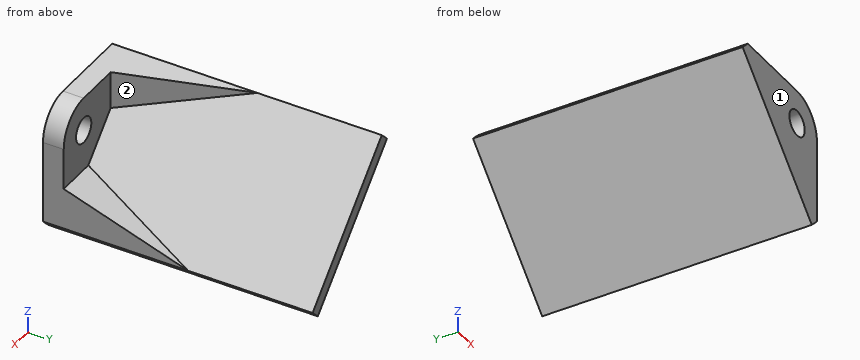
Autodesk Inventor part; units mm, degrees
ref_plane "YZ Plane" through (0, 0, 0) normal (1, 0, 0) x (0, 1, 0)
ref_plane "XZ Plane" through (0, 0, 0) normal (0, 1, 0) x (-1, 0, 0)
ref_plane "XY Plane" through (0, 0, 0) normal (0, 0, 1) x (1, 0, 0)
sketch "스케치1" plane through (0, 0, 0) normal (0, 1, 0) x (-1, 0, 0)
  circle A0 centre (0, 0) radius 3.1
  circle A1 centre (0, 0) radius 8.1
  line L0 (-8.1, 0) -> (-8.1, -20)
  line L1 (0, 8.1) -> (20, 8.1)
  line L2 (20, 8.1) -> (-8.1, -20)
  line L3 (20, 8.1) -> (22.1213, 5.9787)
  line L4 (22.1213, 5.9787) -> (-5.9787, -22.1213)
  line L5 (-5.9787, -22.1213) -> (-8.1, -20)
  dimension "d0" = 6.2
  dimension "d1" = 5
  dimension "d2" = 20
  dimension "d3" = 20
  dimension "d4" = 3
extrude "돌출1" add sketch "스케치1" along normal blind 5
sketch "스케치2" plane through (0, 5, 0) normal (0, 1, 0) x (1, 0, 0)
  line L0 (-22.1213, -5.9787) -> (-20, -8.1)
  line L1 (-20, -8.1) -> (8.1, 20)
  line L2 (5.9787, 22.1213) -> (-22.1213, -5.9787)
  line L3 (8.1, 20) -> (5.9787, 22.1213)
  line L4 (5.9787, 22.1213) -> (-22.1213, -5.9787)
  line L5 (-22.1213, -5.9787) -> (-20, -8.1)
  point P0 (0, 0)
extrude "돌출2" add sketch "스케치2" along normal blind 60
sketch "스케치3" plane through (8.1, 0, 0) normal (1, 0, 0) x (0, 0, -1)
  line L0 (0, 5) -> (20, 5)
  line L1 (10, 5) -> (20, 35)
  line L2 (20, 5) -> (20, 65)
  line L3 (10, 5) -> (20, 5)
  line L4 (20, 5) -> (20, 35)
  point P0 (0, 0)
extrude "돌출3" add sketch "스케치3" against normal blind 10
sketch "스케치4" plane through (-20, 0, 8.1) normal (0, 0, 1) x (1, 0, 0)
  line L0 (18.1, 5) -> (0, 5)
  line L1 (9.05, 5) -> (0, 35)
  line L2 (0, 5) -> (0, 65)
  line L3 (9.05, 5) -> (0, 5)
  line L4 (0, 5) -> (0, 35)
  point P0 (20, 0)
extrude "돌출4" add sketch "스케치4" against normal blind 10
sketch "스케치5" plane through (-22.1213, 0, 5.9787) normal (-0.7071, 0, 0.7071) x (0.7071, 0, 0.7071)
  line L0 (3, 0) -> (0, 0)
  line L1 (0, 35) -> (-4.0711, 35)
  line L2 (0, 0) -> (-4.0711, 0)
  line L3 (-4.0711, 0) -> (-4.0711, 35)
  line L4 (-4.0711, 35) -> (0, 35)
  line L5 (0, 35) -> (0, 0)
  point P0 (11.4146, 0)
extrude "돌출5" cut sketch "스케치5" against normal through all
properties part number "motor_limit_2"
Model file for the job. Use its own axes, mm. Face numbers are marked on the shaded views. A direction names the side the tool comes from. Coordinates: 2 decimals unless noted, no trailing zeros. Write each loop counter-clockwise with the first axis right and the second up, starting at its lowest first coordinate (ties: lowest second). Pieces come first, ordered by that corner, then holes. Notation, with made-up numbers: (39, -11.75) - (45, -11.75) arc R24 cw to (45, 8.25) - close; hole circle Ø6 at (79, 29.5). An arc over 180 degrees is marked (long way). Write each question's results on one line, items separated by ' | '. Start each with the question number.
1) Cut at A-A (y = 33). Write the cut outline in (x, z), then the cut area to 3 significant figures.
2) 3-axis set-ups, long thin cutter, end or side, ignore diameter. For the marked faces 1 and 2: which of +Z, -Z, +X, -X, +Y, -Y reach the whole face in a straight line?
3) Cut at B-B (x = 4). Write the cut outline in (y, z).
4) Flat gauge pins, fed straight in: P1, Ø2, axis at x = -14, y = 38, coming from the -Z side; P2, Ø3, axis at y = 57, z = -5.5, coming from the -X side; P3, Ø5, axis at y = 13.5, z = 1.5, coming from the -X side. Where does each tip first touch, or does it go through?
5) Probe line 1 along Y through (x, z) = (-4, -3); line 2 along Z through (x, y) = (0, 1.65); line 3 along X through (y, z) = (34.5, -21). List the from-to ranges inside material, lowest first. Write a range as from..to.
6) Cut at C-C (z = -8). Write the cut outline in (x, y), then the cut area to 3 significant figures.
7) Cut at D-D (y = 42). Write the cut outline in (x, z).
Returned:
1) outline: (-22.12, 5.98) - (5.98, -22.12) - (8.1, -20) - (8.1, -19.33) - (7.43, -19.33) - (-19.4, 7.5) - (-19.4, 8.1) - (-20, 8.1) - close | area: 120 mm^2
2) face 1: +Z, -Z, +X, -X, -Y | face 2: +Z, +X, +Y
3) outline: (0, -20.14) - (65, -20.14) - (65, -15.9) - (22.7, -15.9) - (5, -10) - (5, 7.04) - (0, 7.04) - close
4) P1: z = -3.14 | P2: x = -12.14 | P3: x = -20.14
5) line 1: 0..5 | line 2: -16.14..-3.1, 3.1..8.1 | line 3: 4.86..7.1
6) outline: (-8.14, 0) - (8.1, 0) - (8.1, 5) - (-3.9, 5) - (-3.9, 65) - (-8.14, 65) - close | area: 336 mm^2
7) outline: (-22.12, 5.98) - (5.98, -22.12) - (8.1, -20) - (-20, 8.1) - close
